Print and shaded views of the part. All mm, measured from the part's lowest x, y and z. A direction names the side the tool comes from. Give positions to 0.01 mm unless a question says otherwise; leave off trailing zeros. Loops run counter-clockwise (first coordinate to the right, second up) from the corner with the lowest first, then second, coordinate; pieces in that order, holes last. Notation, with made-up numbers: M 49,31.5 L 89,31.5 A23 cw 89,43.5 Z; hole C 52.5,71.5 d3. An arc over 180 degrees is marked long. Answer in a Markdown table with one row per item.
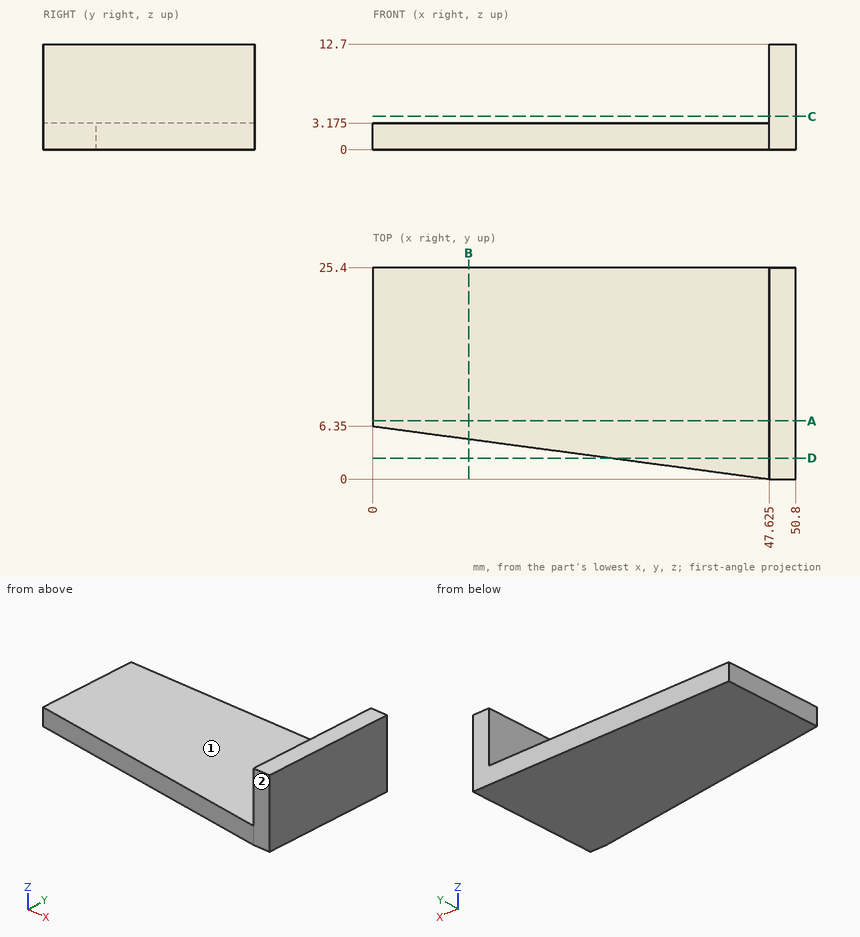
(1) Saw through at D-D, the plane y = 2.5. Give the cut face in (x, z) (3 decimals), and give its area (3 significant figures).
Established:
| item | result |
|---|---|
| outline | M 28.875,0 L 50.8,0 L 50.8,12.7 L 47.625,12.7 L 47.625,3.175 L 28.875,3.175 Z |
| area | 99.9 mm2 |
(2) Saw through at A-A, the plane y = 7. Give the cut face in (x, z) (3 decimals).
Established:
| item | result |
|---|---|
| outline | M 0,0 L 50.8,0 L 50.8,12.7 L 47.625,12.7 L 47.625,3.175 L 0,3.175 Z |
(3) Saw through at B-B, the plane x = 11.5. Give the cut face in (y, z) (3 decimals), and give its area (3 significant figures).
Established:
| item | result |
|---|---|
| outline | M 4.817,0 L 25.4,0 L 25.4,3.175 L 4.817,3.175 Z |
| area | 65.4 mm2 |
(4) Saw through at C-C, the plane z = 4. Give the cut face in (x, y) (3 decimals).
Established:
| item | result |
|---|---|
| outline | M 47.625,0 L 50.8,0 L 50.8,25.4 L 47.625,25.4 Z |
(5) Wall check: L1, parallel to X at y = 2.75, z = 5.25 (3 decimals); L2, parallel to Z at x = 13, y = 19.75 (3 decimals); L3, parallel to Y at x = 40, z = 2.75. Give the ranges that are in metal, low to high.
Established:
| item | result |
|---|---|
| L1 | x = 47.625 to 50.8 |
| L2 | z = 0 to 3.175 |
| L3 | y = 1.02 to 25.4 |
(6) Which spindle directions (+Z, -Z, +X, -X, +Y, -Y) get a long thin tool onto all of the face, cutting with end or side? Do the marked faces 1 and 2. Say none if no direction does.
Established:
| item | result |
|---|---|
| face 1 | +Z, -X, +Y, -Y |
| face 2 | +Z, -Z, +X, -X, -Y |
(7) Flat gauge pins, fed straight in: P1, Ø2, axis at x = 34, y = 19, coming from the +Z side (3 decimals); P2, Ø4, axis at x = 27.5, z = 3, coming from the -Y side; P3, Ø5, axis at y = 16, z = 7, coming from the -X side (3 decimals); P4, Ø4, axis at x = 33, z = 6.5, coming from the +Y side. Where does each tip first touch, or does it go through?
Established:
| item | result |
|---|---|
| P1 | stops at z = 3.175 |
| P2 | stops at y = 2.42 |
| P3 | stops at x = 47.625 |
| P4 | passes through |
